The listing builds one solid part. Answer for the finished solid, in the listing's coordinates (mm). A direction names the side the tool comes from. Give positions to 0.01 mm unless a question says otherwise; leave off trailing zeros. Write each loop counter-clockwise with the first axis right and the second up, starting at its lowest first coordinate (ties: lowest second). Pieces come first, ordered by that corner, then holes.
```python
from build123d import *

# Parameters (mm, degrees)
SKETCH1_W           = 2200
SKETCH1_H           = 600
BOSS_EXTRUDE1_DEPTH = 18
SKETCH2_W           = 18
SKETCH2_H           = 545
BOSS_EXTRUDE2_DEPTH = 742
SKETCH3_W           = 18
SKETCH3_H           = 280
BOSS_EXTRUDE3_DEPTH = 2164


with BuildPart() as part:
    # Sketch1 → Boss-Extrude1 (new body)
    with BuildSketch(Plane(origin=(0, 0, 0), x_dir=(1, 0, 0), z_dir=(0, 1, 0))):
        Rectangle(SKETCH1_W, SKETCH1_H)
    extrude(amount=BOSS_EXTRUDE1_DEPTH)

    # Sketch2 → Boss-Extrude2 (add)
    with BuildSketch(Plane.XZ):
        with Locations((-1091, -27.5)):
            Rectangle(SKETCH2_W, SKETCH2_H)
    boss_extrude2 = extrude(amount=BOSS_EXTRUDE2_DEPTH)

    # Mirror1: Boss-Extrude2 across plane
    add(boss_extrude2.mirror(Plane(origin=(0, 0, 0), x_dir=(0, 0, 1), z_dir=(1, 0, 0))))

    # Sketch3 → Boss-Extrude3 (add)
    with BuildSketch(Plane(origin=(-1082, 0, 0), x_dir=(0, 0, -1), z_dir=(1, 0, 0))):
        with Locations((244, -140)):
            Rectangle(SKETCH3_W, SKETCH3_H)
    extrude(amount=BOSS_EXTRUDE3_DEPTH)


solid = part.part
```
Item 1: A cutting plane is placed at C-C, the plane y = -185. Give the vertices of the cut face in (x, z), plus the area to 3 significant figures.
Conclusion:
outline: (-1100, -300) - (-1082, -300) - (-1082, -253) - (1082, -253) - (1082, -300) - (1100, -300) - (1100, 245) - (1082, 245) - (1082, -235) - (-1082, -235) - (-1082, 245) - (-1100, 245) - close
area: 58,600 mm2
Item 2: Which of the six approach directions +Z, -Z, +X, -X, +Y, -Y give full straight-line access (tool end or side, diameter ignored) to faces 5 (the face through (-15, 0, -277)), 6 (the face through (5, 6, -300))?
Conclusion:
face 5: -Z, -Y
face 6: -Z, +X, -X, +Y, -Y
Item 3: Consider probe 1 along X at (y, z) = (-478, 214); probe 2 along Y at (x, z) = (491, -88); probe 3 along Z at (x, y) = (53, -228). Determine where each line is inside the solid, lowest interval first.
Conclusion:
probe 1: x = -1100 to -1082, 1082 to 1100
probe 2: y = 0 to 18
probe 3: z = -253 to -235
Item 4: A cutting plane is placed at A-A, the plane y = -472. Give the vertices of the cut face in (x, z).
Conclusion:
outline: (-1100, -300) - (-1082, -300) - (-1082, 245) - (-1100, 245) - close; (1082, -300) - (1100, -300) - (1100, 245) - (1082, 245) - close
Item 5: A cutting plane is placed at D-D, the plane x = -218.5. Give the vertices of the cut face in (y, z), plus the area to 3 significant figures.
Conclusion:
outline: (-280, -253) - (0, -253) - (0, -300) - (18, -300) - (18, 300) - (0, 300) - (0, -235) - (-280, -235) - close
area: 15,800 mm2
Item 6: Each of these flat-tipped pins is pushed along its axis until it touches: P1, Ø1.5, axis at x = 709.5, z = 5.5, coming from the -Y side; P2, Ø14.5, axis at x = 1087.5, y = -232, coming from the +Z side; P3, Ø4, axis at x = 183.5, y = -133, coming from the -Z side. Where does it stop, or does it pass through?
Conclusion:
P1: stops at y = 0
P2: stops at z = 245
P3: stops at z = -253
Item 7: A cutting plane is placed at B-B, the plane z = 88.5. Give the vertices of the cut face in (x, y), plus the area to 3 significant figures.
Conclusion:
outline: (-1100, -742) - (-1082, -742) - (-1082, 0) - (1082, 0) - (1082, -742) - (1100, -742) - (1100, 18) - (-1100, 18) - close
area: 66,300 mm2
Item 8: Determine the mould class of faces 1 (the face through (1100, -357, -4)), 2 (the face through (-15, -142, -235)), 3 (the face through (-15, -142, -253)), 4 (the face through (-15, 18, -4)) for opening direction X: pulls with the +X half, pulls with the -X half, needs draft (parallel to the pull), parting line crosses it, or undercut.
Conclusion:
face 1: pulls with the +X half
face 2: undercut
face 3: undercut
face 4: needs draft
